Work out the finished part from the listing and answer in its coordinate system (mm). Coordinates: 2 decimals unless noted, no trailing zeros. Order: outer loops, then holes, each group sorted by start corner. A loop starts at its lowest first (then second) coordinate and runs counter-clockwise, first axis right, second up. Notation, with made-up numbers: (23.25, 49) -> (51.25, 49) arc R13 ccw to (51.25, 63) -> close; hole circle Ø10 at (29, -33.75). An arc over 180 degrees is marked (long way). Write item = value, one per line. Start each with the question number.
Q1. The part is cut by section B-B, the plane y = 1.5. Determine the outline of the cut face in (x, z) (3 decimals).
Q2. A straight line is drawn through the part: L1, parallel to X at y = 0.75, z = 30.5 (3 decimals). Find the intervals that lie inside material, in ascending order. Write a range as from..to.
Q3. The part is cut by section C-C, the plane x = 261. Determine the outline of the cut face in (y, z).
Q4. The part is cut by section A-A, the plane z = 75.5. Determine the outline of the cut face in (x, y) (3 decimals).
Q5. A flat-ended cylindrical pin translates along its axis: pin 1 (1.9 mm diameter, centred on x = 333, y = 3, fed in from -Z). Find the tip coordinate at first contact, or state that the pin passes through.
Autodesk Inventor part; units mm, degrees
ref_plane "YZ Plane" through (0, 0, 0) normal (1, 0, 0) x (0, 1, 0)
ref_plane "XZ Plane" through (0, 0, 0) normal (0, 1, 0) x (-1, 0, 0)
ref_plane "XY Plane" through (0, 0, 0) normal (0, 0, 1) x (1, 0, 0)
sketch "Sketch1" plane through (0, 0, 0) normal (0, 1, 0) x (-1, 0, 0)
  line L0 (0, 0) -> (-660.4, 0)
  line L1 (-660.4, 0) -> (-660.4, 375.2088)
  line L2 (-660.4, 375.2088) -> (0, 375.2088)
  line L3 (0, 375.2088) -> (0, 0)
  dimension "d0" = 660.4
  dimension "d1" = 375.2088
extrude "Extrusion1" add sketch "Sketch1" along normal blind 6.35
sketch "Sketch2" plane through (0, 0, 0) normal (0, -1, 0) x (1, 0, 0)
  line L0 (660.4, 0) -> (0, 0)
  line L1 (225.425, 0) -> (434.975, 0)
  line L2 (434.975, 0) -> (434.975, 190.5)
  line L3 (434.975, 190.5) -> (225.425, 190.5)
  line L4 (225.425, 190.5) -> (225.425, 0)
  line L5 (0, 375.2088) -> (0, 0)
  line L6 (660.4, 0) -> (660.4, 375.2088)
  dimension "d4" = 209.55
  dimension "d5" = 190.5
  dimension "d6" = 225.425
  dimension "d7" = 225.425
extrude "Extrusion2" cut sketch "Sketch2" against normal blind 6.35
properties part number "Electronics Board"
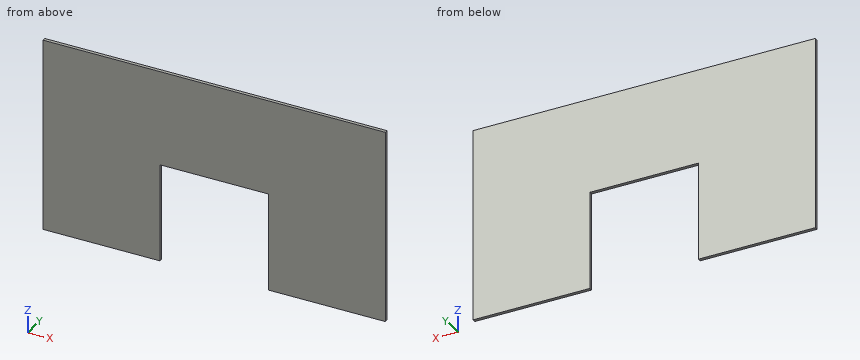
Model answer:
q1.outline = (0, 0) -> (225.425, 0) -> (225.425, 190.5) -> (434.975, 190.5) -> (434.975, 0) -> (660.4, 0) -> (660.4, 375.209) -> (0, 375.209) -> close
q2.L1 = 0..225.425, 434.975..660.4
q3.outline = (0, 190.5) -> (6.35, 190.5) -> (6.35, 375.21) -> (0, 375.21) -> close
q4.outline = (0, 0) -> (225.425, 0) -> (225.425, 6.35) -> (0, 6.35) -> close; (434.975, 0) -> (660.4, 0) -> (660.4, 6.35) -> (434.975, 6.35) -> close
q5.pin_1 = 190.5
